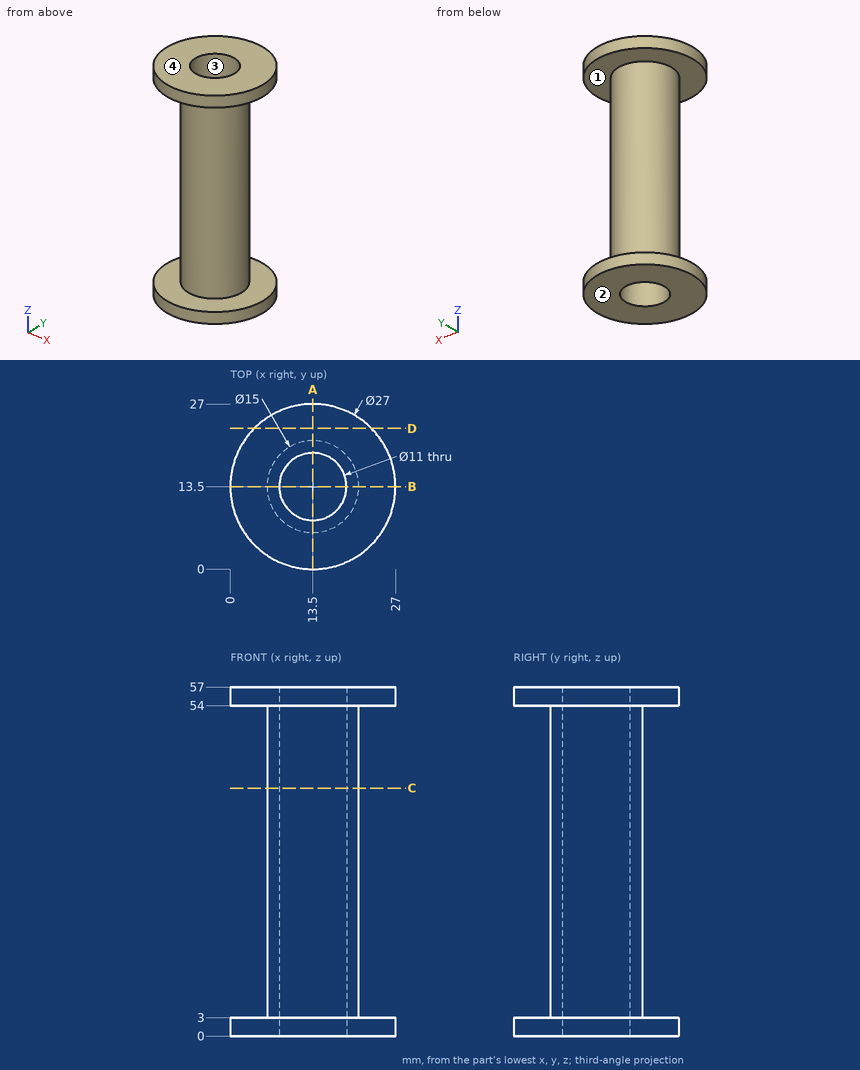
For this review, use the dimensioned drawing (mm, ordinates from the lowest corner) and the shaded views. Give positions to 0.01 mm unless a question says otherwise; leave off trailing zeros. Order: outer loops, then holes, each group sorted by start corner. A loop starts at its lowest first (then second) coordinate and runs counter-clockwise, first axis right, second up.
1) Insertion check: pin 1 (10 mm diameter, centred on x = 13.5, y = 13.5, fed in from -Z); pin 2 (8 mm diameter, centred on x = 8.5, z = 6.5, fed in from +Y); pin 3 (1.5 mm diameter, centred on x = 14.5, z = 33, fed in from -Y); pin 4 (10 mm diameter, centred on x = 20, y = 16, fed in from -Z). Each pin has a flat end and moves straight along its axis. Give the tip position at first contact, or say it passes through.
2) Take a section at A-A (x = 13.5). Give the boundary of the cut face in (y, z), then the cut area to 3 significant figures.
3) Take a section at C-C (z = 40.5). Give the boundary of the cut face in (x, y), then the cut area to 3 significant figures.
4) Take a section at D-D (y = 23). Give the boundary of the cut face in (x, z).
5) The part is to be moulded in two halves that separate along Z. For the marked faces 1, 2, 3 and 4, say which applies: released by +Z, released by -Z, zero draft, split by the parting line, or undercut.
6) Wall thickness on line 1 (Z direction, x = 23.75, y = 7.75); line 2 (X direction, y = 14, z = 51); line 3 (Y direction, x = 15, z = 13.5): over which ranges is each line inside the solid? List them lowest first.
Derived:
1. pin 1: passes through
1. pin 2: stops at y = 26.65
1. pin 3: stops at y = 6
1. pin 4: stops at z = 0
2. outline: (0, 0) - (8, 0) - (8, 57) - (0, 57) - (0, 54) - (6, 54) - (6, 3) - (0, 3) - close; (19, 0) - (27, 0) - (27, 3) - (21, 3) - (21, 54) - (27, 54) - (27, 57) - (19, 57) - close
2. area: 300 mm2
3. outline: circle Ø15 at (13.5, 13.5); hole circle Ø11 at (13.5, 13.5)
3. area: 81.7 mm2
4. outline: (3.91, 0) - (23.09, 0) - (23.09, 3) - (3.91, 3) - close; (3.91, 54) - (23.09, 54) - (23.09, 57) - (3.91, 57) - close
5. face 1: undercut
5. face 2: released by -Z
5. face 3: zero draft
5. face 4: released by +Z
6. line 1: z = 0 to 3, 54 to 57
6. line 2: x = 6.02 to 8.02, 18.98 to 20.98
6. line 3: y = 6.15 to 8.21, 18.79 to 20.85
